Autodesk Inventor part; units mm, degrees
ref_plane "Work Plane1" through (168.275, -1.5875, 2.3038) normal (1, 0, 0) x (0, 1, 0)
ref_plane "Work Plane2" through (0, 0, 0) normal (0, 1, 0) x (1, 0, 0)
ref_plane "XZ Plane" through (0, 0, 0) normal (0, 1, 0) x (-1, 0, 0)
sketch "Sketch1" plane through (0, 0, 0) normal (0, 0, 1) x (1, 0, 0)
  arc A0 (0, 47.625) -> (0, -47.625) centre (0, 0) ccw
  line L0 (-47.625, 0) -> (384.175, 0) construction
  arc A1 (336.55, -47.625) -> (336.55, 47.625) centre (336.55, 0) ccw
  line L1 (0, 47.625) -> (336.55, 47.625)
  line L2 (336.55, -47.625) -> (0, -47.625)
  dimension "d0" = 95.25
  dimension "d1" = 431.8
  dimension "d2" = 95.25
extrude "Extrusion1" add sketch "Sketch1" along normal blind 2.3038
hole "Hole1" at (0, 0, 2.3038) direction (0, 0, -1) diameter 8 end through all
hole "Hole2" at (336.55, 0, 2.3038) direction (0, 0, -1) diameter 8 end through all
sketch "Sketch2" plane through (0, 0, 2.3038) normal (0, 0, 1) x (1, 0, 0)
  circle A0 centre (336.55, 0) radius 4
  circle A1 centre (0, 0) radius 4
  line L0 (336.55, 0) -> (0, 0) construction
  line L1 (168.275, 0) -> (168.275, -1.5875)
  point P0 (0, 0)
  dimension "d23" = 1.5875
hole "Hole3" at (168.275, -1.5875, 2.3038) direction (0, 0, -1) diameter 8 end through all
sketch "Sketch4" plane through (0, 0, 2.3038) normal (0, 0, 1) x (1, 0, 0)
  line L0 (336.55, 47.625) -> (0, 47.625)
  line L1 (0, -47.625) -> (336.55, -47.625)
  line L2 (168.275, 47.625) -> (168.275, -47.625)
  line L3 (168.275, 0) -> (238.125, 0)
  line L4 (168.275, 0) -> (98.425, 0)
  point P0 (0, 0)
  dimension "d41" = 69.85
  dimension "d42" = 69.85
hole "Hole5" at (98.425, 0, 2.3038) at (238.125, 0, 2.3038) direction (0, 0, -1) diameter 38.1 end through all
sketch "Sketch5" plane through (0, 0, 0) normal (0, 0, -1) x (-1, 0, 0)
  line L0 (-89.425, 29) -> (-89.425, 26.5)
  arc A0 (-89.925, 26) -> (-89.425, 26.5) centre (-89.925, 26.5) ccw
  line L1 (-94.925, 26) -> (-89.925, 26)
  arc A1 (-94.925, 26) -> (-95.425, 25.5) centre (-94.925, 25.5) ccw
  line L2 (-95.425, 19) -> (-95.425, 25.5)
  arc A2 (-95.925, 18.5) -> (-95.425, 19) centre (-95.925, 19) ccw
  line L3 (-98.425, 18.5) -> (-95.925, 18.5)
  arc A3 (-98.425, 18.5) -> (-98.425, -18.5) centre (-98.425, 0) ccw
  line L4 (-95.925, -18.5) -> (-98.425, -18.5)
  arc A4 (-95.425, -19) -> (-95.925, -18.5) centre (-95.925, -19) ccw
  line L5 (-95.425, -25.5) -> (-95.425, -19)
  arc A5 (-95.425, -25.5) -> (-94.925, -26) centre (-94.925, -25.5) ccw
  line L6 (-89.925, -26) -> (-94.925, -26)
  arc A6 (-89.425, -26.5) -> (-89.925, -26) centre (-89.925, -26.5) ccw
  line L7 (-89.425, -26.5) -> (-89.425, -29)
  arc A7 (-92.425, -32) -> (-89.425, -29) centre (-92.425, -29) ccw
  line L8 (-92.425, -32) -> (-118.425, -32)
  arc A8 (-121.425, -29) -> (-118.425, -32) centre (-118.425, -29) ccw
  line L9 (-121.425, -29) -> (-121.425, 29)
  arc A9 (-118.425, 32) -> (-121.425, 29) centre (-118.425, 29) ccw
  line L10 (-118.425, 32) -> (-92.425, 32)
  arc A10 (-89.425, 29) -> (-92.425, 32) centre (-92.425, 29) ccw
  arc A11 (-105.425, 25.85) -> (-105.425, 22.15) centre (-105.425, 24) ccw
  arc A12 (-105.425, 22.15) -> (-105.425, 25.85) centre (-105.425, 24) ccw
  arc A13 (-105.425, -22.15) -> (-105.425, -25.85) centre (-105.425, -24) ccw
  arc A14 (-105.425, -25.85) -> (-105.425, -22.15) centre (-105.425, -24) ccw
  line L11 (-247.125, -29) -> (-247.125, -26.5)
  arc A15 (-246.625, -26) -> (-247.125, -26.5) centre (-246.625, -26.5) ccw
  line L12 (-241.625, -26) -> (-246.625, -26)
  arc A16 (-241.625, -26) -> (-241.125, -25.5) centre (-241.625, -25.5) ccw
  line L13 (-241.125, -19) -> (-241.125, -25.5)
  arc A17 (-240.625, -18.5) -> (-241.125, -19) centre (-240.625, -19) ccw
  line L14 (-238.125, -18.5) -> (-240.625, -18.5)
  arc A18 (-238.125, -18.5) -> (-238.125, 18.5) centre (-238.125, 0) ccw
  line L15 (-240.625, 18.5) -> (-238.125, 18.5)
  arc A19 (-241.125, 19) -> (-240.625, 18.5) centre (-240.625, 19) ccw
  line L16 (-241.125, 25.5) -> (-241.125, 19)
  arc A20 (-241.125, 25.5) -> (-241.625, 26) centre (-241.625, 25.5) ccw
  line L17 (-246.625, 26) -> (-241.625, 26)
  arc A21 (-247.125, 26.5) -> (-246.625, 26) centre (-246.625, 26.5) ccw
  line L18 (-247.125, 26.5) -> (-247.125, 29)
  arc A22 (-244.125, 32) -> (-247.125, 29) centre (-244.125, 29) ccw
  line L19 (-244.125, 32) -> (-218.125, 32)
  arc A23 (-215.125, 29) -> (-218.125, 32) centre (-218.125, 29) ccw
  line L20 (-215.125, 29) -> (-215.125, -29)
  arc A24 (-218.125, -32) -> (-215.125, -29) centre (-218.125, -29) ccw
  line L21 (-218.125, -32) -> (-244.125, -32)
  arc A25 (-247.125, -29) -> (-244.125, -32) centre (-244.125, -29) ccw
  arc A26 (-231.125, -25.85) -> (-231.125, -22.15) centre (-231.125, -24) ccw
  arc A27 (-231.125, -22.15) -> (-231.125, -25.85) centre (-231.125, -24) ccw
  arc A28 (-231.125, 22.15) -> (-231.125, 25.85) centre (-231.125, 24) ccw
  arc A29 (-231.125, 25.85) -> (-231.125, 22.15) centre (-231.125, 24) ccw
  point P0 (0, 0)
extrude "Extrusion2" cut sketch "Sketch5" against normal through all contours A12 A11 | A14 A13 | A27 A26 | A29 A28
ref_plane "Work Plane1" through (168.275, -1.5875, 2.3038) normal (1, 0, 0) x (0, 1, 0)
sketch "Sketch7" plane through (0, 0, 0) normal (0, 0, -1) x (-1, 0, 0)
  point P0 (0, 0)
sketch "Sketch8" plane through (0, 0, 2.3038) normal (0, 0, 1) x (1, 0, 0)
  arc A0 (286.775, -21.025) -> (284.775, -23.025) centre (286.775, -23.025) ccw
  line L0 (284.775, -45.625) -> (284.775, -23.025)
  line L1 (294.275, -45.625) -> (284.775, -45.625)
  line L2 (294.275, -45.625) -> (294.275, -23.025)
  arc A1 (294.275, -23.025) -> (292.275, -21.025) centre (292.275, -23.025) ccw
  line L3 (292.275, -21.025) -> (286.775, -21.025)
  circle A2 centre (288.025, -36.025) radius 1.85
  circle A3 centre (288.025, -26.025) radius 1.85
  arc A4 (243.775, -23.025) -> (241.775, -21.025) centre (241.775, -23.025) ccw
  line L4 (241.775, -21.025) -> (236.275, -21.025)
  arc A5 (236.275, -21.025) -> (234.275, -23.025) centre (236.275, -23.025) ccw
  line L5 (234.275, -45.625) -> (234.275, -23.025)
  line L6 (243.775, -45.625) -> (234.275, -45.625)
  line L7 (243.775, -45.625) -> (243.775, -23.025)
  circle A6 centre (240.525, -36.025) radius 1.85
  circle A7 centre (240.525, -26.025) radius 1.85
  arc A8 (94.775, -21.025) -> (92.775, -23.025) centre (94.775, -23.025) ccw
  line L8 (92.775, -45.625) -> (92.775, -23.025)
  line L9 (102.275, -45.625) -> (92.775, -45.625)
  line L10 (102.275, -45.625) -> (102.275, -23.025)
  arc A9 (102.275, -23.025) -> (100.275, -21.025) centre (100.275, -23.025) ccw
  line L11 (100.275, -21.025) -> (94.775, -21.025)
  circle A10 centre (96.025, -36.025) radius 1.85
  circle A11 centre (96.025, -26.025) radius 1.85
  arc A12 (51.775, -23.025) -> (49.775, -21.025) centre (49.775, -23.025) ccw
  line L12 (49.775, -21.025) -> (44.275, -21.025)
  arc A13 (44.275, -21.025) -> (42.275, -23.025) centre (44.275, -23.025) ccw
  line L13 (42.275, -45.625) -> (42.275, -23.025)
  line L14 (51.775, -45.625) -> (42.275, -45.625)
  line L15 (51.775, -45.625) -> (51.775, -23.025)
  circle A14 centre (48.525, -36.025) radius 1.85
  circle A15 centre (48.525, -26.025) radius 1.85
  point P0 (0, 0)
extrude "Extrusion4" cut sketch "Sketch8" against normal through all contours A2 | A3 | A6 | A7 | A10 | A11 | A14 | A15
sketch "Sketch9" plane through (0, 0, 2.3038) normal (0, 0, 1) x (1, 0, 0)
  line L0 (0, -47.625) -> (336.55, -47.625)
  line L1 (54.775, -49.225) -> (54.775, -46.025)
  line L2 (54.775, -46.025) -> (89.775, -46.025)
  line L3 (89.775, -46.025) -> (89.775, -49.225)
  line L4 (54.775, -47.625) -> (89.775, -47.625)
  point P0 (0, 0)
  dimension "d57" = 3.2
extrude "Extrusion5" cut sketch "Sketch9" against normal through all
mirror "Mirror2" about plane through (168.275, -1.5875, 2.3038) normal (1, 0, 0) of "Extrusion5"
ref_plane "Work Plane2" through (0, 0, 0) normal (0, 1, 0) x (1, 0, 0)
mirror "Mirror3" about plane through (0, 0, 0) normal (0, 1, 0) of "Extrusion4", "Extrusion5", "Mirror2"
properties part number "SidePlate" material "Aluminum 6061"
Can you work these out from the model? Positions are in its coordinate system, mm. Coordinates: 2 decimals unless noted, no trailing zeros. Loops run counter-clockwise (first coordinate to the right, second up) from the corner with the lowest first, then second, coordinate; pieces in that order, holes last. Notation, with made-up numbers: (65.5, 46) - (112.5, 46) arc R17 ccw to (112.5, 74) - close; hole circle Ø9 at (-13.75, 9.25). An arc over 180 degrees is marked (long way). Use a Markdown table: item, result.
Item 1: We'd pull the mould along X, two halves only. Please class faces 1 (the face through (-47.613, -1.047, 1.136)), 2 (the face through (165, -10, 2.304)), 3 (the face through (219.237, 2.48, 1.136)): released by +X, released by -X, zero draft, split by the parting line, or undercut.
Numbers:
| item | result |
|---|---|
| face 1 | released by -X |
| face 2 | zero draft |
| face 3 | undercut |
Item 2: I want a section at B-B on z = 1.5. Give the number of separate pieces and of enclosed holes in the cut face, and give its area (3 significant figures).
Numbers:
| item | result |
|---|---|
| separate pieces | 1 |
| enclosed holes | 25 |
| area | 36,300 mm2 |
Item 3: I want a section at A-A on x = 267. Please give me the cut outline in (y, z) (3 decimals), and give its area (3 significant figures).
Numbers:
| item | result |
|---|---|
| outline | (-46.025, 0) - (46.025, 0) - (46.025, 2.304) - (-46.025, 2.304) - close |
| area | 212 mm2 |
Item 4: Will these pins go through, and if not, where does the flat tip stop? pin 1 (0.7 mm diameter, centred on x = 265.5, z = 1.5, fed in from +Y) (3 decimals); pin 2 (6 mm diameter, centred on x = 48.525, y = 36.025, fed in from -Z); pin 3 (3.5 mm diameter, centred on x = 105.425, y = 24, fed in from -Z); pin 4 (1 mm diameter, centred on y = -25.5, z = 1.5, fed in from -X).
Numbers:
| item | result |
|---|---|
| pin 1 | stops at y = 46.025 |
| pin 2 | stops at z = 0 |
| pin 3 | passes through |
| pin 4 | stops at x = -40.54 |
Item 5: If I drill on probe 1 along X at (y, z) = (16, 2); probe 2 along X at (y, z) = (-27, 0.1); probe 3 along X at (y, z) = (15, 1), over which ranges is the centre line in solid material (lowest first)? Write a range as from..to.
Numbers:
| item | result |
|---|---|
| probe 1 | x = -44.86..88.09, 108.76..227.79, 248.46..381.41 |
| probe 2 | x = -39.23..46.95, 50.1..94.45, 97.6..238.95, 242.1..286.45, 289.6..375.78 |
| probe 3 | x = -45.2..86.68, 110.17..226.38, 249.87..381.75 |
